Autodesk Inventor part; units mm, degrees
ref_plane "Work Plane1" through (0, 4, 0) normal (0, 1, 0) x (1, 0, 0)
ref_plane "YZ Plane" through (0, 0, 0) normal (1, 0, 0) x (0, 1, 0)
ref_plane "XZ Plane" through (0, 0, 0) normal (0, 1, 0) x (-1, 0, 0)
sketch "Sketch2" plane through (0, 0, 0) normal (0, 1, 0) x (-1, 0, 0)
  line L0 (15, 26) -> (-15, 26)
  line L1 (-15, 26) -> (-15, -26)
  line L2 (-15, -26) -> (15, -26)
  line L3 (15, -26) -> (15, 26)
  line L4 (0, 0) -> (0, -26) construction
  line L5 (0, 0) -> (0, 26) construction
  line L6 (0, 0) -> (15, 0) construction
  line L7 (0, 0) -> (-15, 0) construction
  dimension "d45" = 30
  dimension "d46" = 52
extrude "Main Body Sketch" add sketch "Sketch2" along normal blind 4
ref_plane "Work Plane1" through (0, 4, 0) normal (0, 1, 0) x (1, 0, 0)
sketch "Sketch4" plane through (0, 4, 0) normal (0, 1, 0) x (1, 0, 0)
  circle A0 centre (0, -18) radius 4.8537
  line L0 (15, 26) -> (-15, 26)
  line L1 (-15, 26) -> (-15, -26)
  circle A1 centre (5, 14.5) radius 2.15
  circle A2 centre (-5, 14.5) radius 2.15
  line L2 (15, -26) -> (15, 26)
  dimension "d84" = 44
  dimension "d85" = 30
  dimension "d86" = 15
  dimension "d87" = 4.3
  dimension "d88" = 4.3
  dimension "d89" = 10
  dimension "d90" = 10
  dimension "d91" = 11.5
  dimension "d92" = 11.5
extrude "Holes Cuts" cut sketch "Sketch4" against normal up to surface (4 mm away)
fillet "Fillet12" radius 4 2 edges at (-15, 2, -26) (15, 2, -26)
fillet "Fillet12" radius 15 2 edges at (15, 2, 26) (-15, 2, 26)
fillet "Fillet13" radius 1 12 edges at (10.6066, 4, 21.6066) (15, 4, -5.5) (13.8285, 4, -24.8285) (0, 4, -26) (-13.8285, 4, -24.8285) (-15, 4, -5.5) (15, 0, -5.5) (13.8285, 0, -24.8285) (0, 0, -26) (-13.8285, 0, -24.8285) (-15, 0, -5.5) (10.6066, 0, 21.6066)
equation "\"d46\" = AH"
equation "\"AH\" = 52"
equation "\"d57\" = TMROL"
equation "\"BD\" = 4"
properties part number "Side Attatchment"
Here's how the part is built. I have some questions about the finished solid (model axes, mm). Round coordinates to 2 decimals unless told otherwise and drop trailing zeros. Loops run counter-clockwise (first coordinate to the right, second up) from the corner with the lowest first, then second, coordinate; pieces in that order, holes last. Notation, with made-up numbers: M 32,-39.75 L 70,-39.75 A20 ccw 70,-27.75 Z; hole C 6.25,47.5 d2. An arc over 180 degrees is marked long. Write each question's results on one line, items separated by ' | '. Start each with the question number.
(1) If I drill on probe 1 along X at (y, z) = (0.9, -14.5); probe 2 along Z at (x, y) = (0, 2); probe 3 along Z at (x, y) = (1.5, 2.95), over which ranges is the centre line in solid material (lowest first)? Write a range as from..to.
(2) I want a section at A-A (z = -14.5). Please give me the cut outline in (x, y).
(3) Thinking about a two-plate mould opening in X: for faces 1 (the cylindrical face through (-13.797, 2.014, -24.859)), 2 (the cylindrical face through (-0.154, 3.715, -25.699)), 3 (the cylindrical face through (-5.47, 2.03, -12.4)), which applies, pulls with the +X half, pulls with the -X half, needs draft (parallel to the pull), parting line crosses it, or undercut?
(4) Will these pins go through, and if not, where does the flat tip stop? P1, Ø8, axis at x = 0, z = 18, coming from the -Y side; P2, Ø12, axis at x = -3, z = -15, coming from the +Y side.
Solved:
1) probe 1: x = -14.99..-7.15, -2.85..2.85, 7.15..14.99 | probe 2: z = -26..13.15, 22.85..26 | probe 3: z = -26..13.38, 22.62..25.92
2) outline: M -15,1 A1 ccw -14,0 L -7.15,0 L -7.15,4 L -14,4 A1 ccw -15,3 Z; M -2.85,0 L 2.85,0 L 2.85,4 L -2.85,4 Z; M 7.15,0 L 14,0 A1 ccw 15,1 L 15,3 A1 ccw 14,4 L 7.15,4 Z
3) face 1: pulls with the -X half | face 2: needs draft | face 3: undercut
4) P1: passes through | P2: stops at y = 4
